from build123d import *

# Parameters (mm, degrees)
F0_R            = 11.1
F1_DEPTH        = 7
F1_COPIES_COUNT = 3


# Not quite as in the source:
# - a pattern or mirror of a feature is missing from the dataset's text; its kind, count and spacing are read off the source's solid


with BuildPart() as f1:
    # F0 (on Top) → F1 (new body)
    with BuildSketch(Plane.XY):
        with BuildLine():
            ThreePointArc((14.0864100033, 29.3810870676), (14.0966020914, 29.690468941), (14.1, 30))
            ThreePointArc((14.1, 30), (12.9626271297, 35.5479994499), (9.7340002984, 40.200943005))
            ThreePointArc((9.7340002984, 40.200943005), (0, 44.1), (-9.7340002984, 40.200943005))
            ThreePointArc((-9.7340002984, 40.200943005), (-13.0812960888, 35.2620996416), (-14.0864100033, 29.3810870676))
            ThreePointArc((-14.0864100033, 29.3810870676), (0, 15.9), (14.0864100033, 29.3810870676))
        make_face()
        with Locations((0, 30)):
            Circle(F0_R, mode=Mode.SUBTRACT)
        with BuildLine():
            ThreePointArc((9.7340002984, 40.200943005), (12.9626271297, 35.5479994499), (14.1, 30))
            ThreePointArc((14.1, 30), (14.0966020914, 29.690468941), (14.0864100033, 29.3810870676))
            ThreePointArc((14.0864100033, 29.3810870676), (17.5199942586, 15), (14.0864100033, 0.6189129324))
            ThreePointArc((14.0864100033, 0.6189129324), (14.0966020914, 0.309531059), (14.1, 0))
            ThreePointArc((14.1, 0), (12.9626271297, -5.5479994499), (9.7340002984, -10.200943005))
            ThreePointArc((9.7340002984, -10.200943005), (20.5199942586, 15), (9.7340002984, 40.200943005))
        make_face()
        with BuildLine():
            ThreePointArc((-9.7340002984, -10.200943005), (0, -14.1), (9.7340002984, -10.200943005))
            ThreePointArc((9.7340002984, -10.200943005), (12.9626271297, -5.5479994499), (14.1, 0))
            ThreePointArc((14.1, 0), (14.0966020914, 0.309531059), (14.0864100033, 0.6189129324))
            ThreePointArc((14.0864100033, 0.6189129324), (0, 14.1), (-14.0864100033, 0.6189129324))
            ThreePointArc((-14.0864100033, 0.6189129324), (-13.0812960888, -5.2620996416), (-9.7340002984, -10.200943005))
        make_face()
        Circle(F0_R, mode=Mode.SUBTRACT)
        with BuildLine():
            ThreePointArc((-14.0864100033, 29.3810870676), (-13.0812960888, 35.2620996416), (-9.7340002984, 40.200943005))
            ThreePointArc((-9.7340002984, 40.200943005), (-20.5199942586, 15), (-9.7340002984, -10.200943005))
            ThreePointArc((-9.7340002984, -10.200943005), (-13.0812960888, -5.2620996416), (-14.0864100033, 0.6189129324))
            ThreePointArc((-14.0864100033, 0.6189129324), (-17.5199942586, 15), (-14.0864100033, 29.3810870676))
        make_face()
    extrude(amount=F1_DEPTH)

    # F1_copies: F1 ×3 about axis
    f1_copies_axis = Axis((0, 0, 0), (0, 0, 1))


with BuildPart() as f1_1:
    add(f1.part)
    for i in range(1, F1_COPIES_COUNT):
        add(f1.part.rotate(f1_copies_axis, i * 360 / F1_COPIES_COUNT))


solid = f1_1.part
For this review, take the finished solid that the model builds, in its own axes (mm). Round coordinates to 2 decimals unless told otherwise and drop trailing zeros. Loops run counter-clockwise (first coordinate to the right, second up) from the corner with the lowest first, then second, coordinate; pieces in that order, holes last. Notation, with made-up numbers: (26.5, 86) - (53.5, 86) arc R20 cw to (53.5, 100) - close; hole circle Ø3 at (6, -34). An arc over 180 degrees is marked (long way). Use one line per item in the form item = value.
Item 1: Consider section B-B on x = -35. Write out the cut boundary in (y, z), then the cut area to 3 significant figures.
Answers:
outline = (-25.84, 0) - (-21.47, 0) - (-21.47, 7) - (-25.84, 7) - close; (-8.53, 0) - (-0.85, 0) - (-0.85, 7) - (-8.53, 7) - close
area = 84.3 mm^2
Item 2: For line 1 (Y direction, x = 26.5, z = 5.25); line 2 (X direction, y = 0, z = 4.5); line 3 (Y direction, x = -7, z = 1), list the stretches that pass through material, from the lowest coordinate up.
Answers:
line_1 = -29.35 to -26.09, -3.91 to -0.91, 4.32 to 8.14
line_2 = -34.43 to -30.68, -17.12 to -11.1, 11.1 to 17.12, 30.68 to 34.43
line_3 = -27.36 to -24.1, -16.93 to -8.61, 8.61 to 14.92, 17.76 to 21.39, 38.61 to 42.24
Item 3: Consider section C-C on x = -24.5. Write out the cut boundary in (y, z).
Answers:
outline = (-29.66, 0) - (-26, 0) - (-26, 7) - (-29.66, 7) - close; (-4, 0) - (-0.98, 0) - (-0.98, 7) - (-4, 7) - close; (5.89, 0) - (9.51, 0) - (9.51, 7) - (5.89, 7) - close
Item 4: Consider section D-D on y = 2.5. Write out the cut boundary in (x, z).
Answers:
outline = (-32.51, 0) - (-28.46, 0) - (-28.46, 7) - (-32.51, 7) - close; (-18.2, 0) - (-14.96, 0) - (-14.96, 7) - (-18.2, 7) - close; (-13.88, 0) - (-10.81, 0) - (-10.81, 7) - (-13.88, 7) - close; (10.81, 0) - (13.88, 0) - (13.88, 7) - (10.81, 7) - close; (14.96, 0) - (18.2, 0) - (18.2, 7) - (14.96, 7) - close; (28.46, 0) - (32.51, 0) - (32.51, 7) - (28.46, 7) - close
Item 5: Clearance check with flat-ended pins moving along their axes: P1, Ø12, axis at x = -14, y = 3.5, coming from the +Z side; P2, Ø1.5, axis at x = 14.5, z = 4, coming from the +Y side; P3, Ø1.5, axis at x = -26, z = 4.5, coming from the +Y side. State where each tip first meets the part, or that it passes through.
Answers:
P1 = 7
P2 = 35.64
P3 = 9.02
Item 6: Consider section A-A on y = -15. Write out the cut boundary in (x, z).
Answers:
outline = (-40.08, 0) - (-37.08, 0) - (-37.08, 7) - (-40.08, 7) - close; (-14.88, 0) - (-11.88, 0) - (-11.88, 7) - (-14.88, 7) - close; (-8.45, 0) - (-4.7, 0) - (-4.7, 7) - (-8.45, 7) - close; (4.7, 0) - (8.45, 0) - (8.45, 7) - (4.7, 7) - close; (11.88, 0) - (14.88, 0) - (14.88, 7) - (11.88, 7) - close; (37.08, 0) - (40.08, 0) - (40.08, 7) - (37.08, 7) - close
Item 7: Mouldability with a two-part tool opening along X and no side actions: class faces 1 (the cylindrical face through (0.2, 44.1, 3.5)), 2 (the flat face through (-9, 9, 7)), 3 (the cylindrical face through (32.85, 2.09, 3.45)), 4 (the cylindrical face through (14.183, -29.423, 3.451)) as +X half, -X half, draft (parallel to the pull), parting line (faces both ways), or undercut.
Answers:
face_1 = parting line
face_2 = draft
face_3 = +X half
face_4 = undercut
